```python
from build123d import *
from build123d.topology import SkipClean

# Parameters (mm, degrees)
SCHIZZO2_W            = 65.8
SCHIZZO2_H            = 15.8
FRONT_DEPTH           = 1.5
INNER_DEPTH           = 34
FRONT_CLEARANCE_DEPTH = 1
BACK_START            = -1
BACK_CLEARANCE_DEPTH  = 1
SCHIZZO7_W            = 65.8
SCHIZZO7_H            = 15.8
BACK_DEPTH            = 2
SCHIZZO9_W            = 65.8
SCHIZZO9_H            = 15.8
BACK_CLOSING_DEPTH    = 1


with BuildPart() as part:
    # Schizzo2 → Front (new, symmetric)
    with BuildSketch(Plane.XY):
        Rectangle(SCHIZZO2_W, SCHIZZO2_H)
        with BuildLine():
            Line((-27.25, 5.4), (-22.75, 5.4))
            Line((-22.75, 5.4), (-21.014451547, 2.089354811))
            ThreePointArc((-21.014451547, 2.089354811), (-25, -4.5), (-28.985548453, 2.089354811))
            Line((-28.985548453, 2.089354811), (-27.25, 5.4))
        make_face(mode=Mode.SUBTRACT)
        with BuildLine():
            Line((27.25, 5.4), (22.75, 5.4))
            Line((22.75, 5.4), (21.014451547, 2.089354811))
            ThreePointArc((21.014451547, 2.089354811), (25, -4.5), (28.985548453, 2.089354811))
            Line((28.985548453, 2.089354811), (27.25, 5.4))
        make_face(mode=Mode.SUBTRACT)
    extrude(amount=FRONT_DEPTH, both=True)

    # Schizzo5 → Inner (add)
    with SkipClean():  # the faces are left unmerged after this step: merging them gives an invalid solid
        with BuildSketch(Plane(origin=(0, 0, -1.5), x_dir=(-1, 0, 0), z_dir=(0, 0, -1))):
            with BuildLine():
                Line((-25, -7.9), (-27.35991702, -7.9))
                Line((-27.35991702, -7.9), (-28.2, -1.922498999))
                Line((-28.2, -1.922498999), (-27.5, -1.922498999))
                ThreePointArc((-27.5, -1.922498999), (-25, -2.8), (-22.5, -1.922498999))
                Line((-22.5, -1.922498999), (-21.5, -1.922498999))
                Line((-21.5, -1.922498999), (-21.5, -4.422498999))
                Line((-21.5, -4.422498999), (-21.15, -4.422498999))
                Line((-21.15, -4.422498999), (-20.726632237, -1.410080834))
                ThreePointArc((-20.726632237, -1.410080834), (-20.515143622, 0.368867555), (-21.014451547, 2.089354811))
                Line((-21.014451547, 2.089354811), (-22.75, 5.4))
                Line((-22.75, 5.4), (-27.25, 5.4))
                Line((-27.25, 5.4), (-28.985548453, 2.089354811))
                ThreePointArc((-28.985548453, 2.089354811), (-29.485161475, 0.365139069), (-29.271017396, -1.417183969))
                Line((-29.271017396, -1.417183969), (-28.35991702, -7.9))
                Line((-28.35991702, -7.9), (-32.9, -7.9))
                Line((-32.9, -7.9), (-32.9, 7.9))
                Line((-32.9, 7.9), (32.9, 7.9))
                Line((32.9, 7.9), (32.9, -7.9))
                Line((32.9, -7.9), (28.35991702, -7.9))
                Line((28.35991702, -7.9), (29.271017396, -1.417183969))
                ThreePointArc((29.271017396, -1.417183969), (29.485161475, 0.365139069), (28.985548453, 2.089354811))
                Line((28.985548453, 2.089354811), (27.25, 5.4))
                Line((27.25, 5.4), (22.75, 5.4))
                Line((22.75, 5.4), (21.014451547, 2.089354811))
                ThreePointArc((21.014451547, 2.089354811), (20.515143622, 0.368867555), (20.726632237, -1.410080834))
                Line((20.726632237, -1.410080834), (21.15, -4.422498999))
                Line((21.15, -4.422498999), (21.5, -4.422498999))
                Line((21.5, -4.422498999), (21.5, -1.922498999))
                Line((21.5, -1.922498999), (22.5, -1.922498999))
                ThreePointArc((22.5, -1.922498999), (25, -2.8), (27.5, -1.922498999))
                Line((27.5, -1.922498999), (28.2, -1.922498999))
                Line((28.2, -1.922498999), (27.35991702, -7.9))
                Line((27.35991702, -7.9), (25, -7.9))
                Line((25, -7.9), (21.638730893, -7.9))
                Line((21.638730893, -7.9), (-21.638730893, -7.9))
                Line((-21.638730893, -7.9), (-25, -7.9))
            make_face()
        extrude(amount=INNER_DEPTH)

    # Schizzo13 → Front clearance (cut)
    with BuildSketch(Plane.XY.offset(-1.5)):
        with BuildLine():
            Line((-21.5, -2.828427125), (-21.5, -4.422498999))
            Line((-21.5, -4.422498999), (-21.15, -4.422498999))
            Line((-21.15, -4.422498999), (-21.155384602, -4.46081243))
            Line((-21.155384602, -4.46081243), (-21.638730893, -7.9))
            Line((-21.638730893, -7.9), (-27.35991702, -7.9))
            Line((-27.35991702, -7.9), (-27.998629063, -3.355327665))
            Line((-27.998629063, -3.355327665), (-28.2, -1.922498999))
            Line((-28.2, -1.922498999), (-27.5, -1.922498999))
            ThreePointArc((-27.5, -1.922498999), (-25, -2.8), (-22.5, -1.922498999))
            Line((-22.5, -1.922498999), (-21.5, -1.922498999))
            Line((-21.5, -1.922498999), (-21.5, -2.828427125))
        make_face()
        with BuildLine():
            Line((21.155384602, -4.46081243), (21.638730893, -7.9))
            Line((21.638730893, -7.9), (27.35991702, -7.9))
            Line((27.35991702, -7.9), (27.998629063, -3.355327665))
            Line((27.998629063, -3.355327665), (28.2, -1.922498999))
            Line((28.2, -1.922498999), (27.5, -1.922498999))
            ThreePointArc((27.5, -1.922498999), (25, -2.8), (22.5, -1.922498999))
            Line((22.5, -1.922498999), (21.5, -1.922498999))
            Line((21.5, -1.922498999), (21.5, -2.828427125))
            Line((21.5, -2.828427125), (21.5, -4.422498999))
            Line((21.5, -4.422498999), (21.15, -4.422498999))
            Line((21.15, -4.422498999), (21.155384602, -4.46081243))
        make_face()
    extrude(amount=-FRONT_CLEARANCE_DEPTH, mode=Mode.SUBTRACT)

    # Schizzo12 → Back clearance (cut)
    with BuildSketch(Plane(origin=(0, 0, -35.5), x_dir=(-1, 0, 0), z_dir=(0, 0, -1)).offset(BACK_START)):
        with BuildLine():
            Line((21.5, -1.922498999), (21.5, -4.422498999))
            Line((21.5, -4.422498999), (21.15, -4.422498999))
            Line((21.15, -4.422498999), (21.638730893, -7.9))
            Line((21.638730893, -7.9), (27.35991702, -7.9))
            Line((27.35991702, -7.9), (28.2, -1.922498999))
            Line((28.2, -1.922498999), (27.5, -1.922498999))
            ThreePointArc((27.5, -1.922498999), (25, -2.8), (22.5, -1.922498999))
            Line((22.5, -1.922498999), (21.5, -1.922498999))
        make_face()
        with BuildLine():
            Line((-27.35991702, -7.9), (-21.638730893, -7.9))
            Line((-21.638730893, -7.9), (-21.15, -4.422498999))
            Line((-21.15, -4.422498999), (-21.5, -4.422498999))
            Line((-21.5, -4.422498999), (-21.5, -1.922498999))
            Line((-21.5, -1.922498999), (-22.5, -1.922498999))
            ThreePointArc((-22.5, -1.922498999), (-25, -2.8), (-27.5, -1.922498999))
            Line((-27.5, -1.922498999), (-28.2, -1.922498999))
            Line((-28.2, -1.922498999), (-27.35991702, -7.9))
        make_face()
    extrude(amount=BACK_CLEARANCE_DEPTH, mode=Mode.SUBTRACT)

    # Schizzo7 → Back (add)
    with BuildSketch(Plane(origin=(0, 0, -35.5), x_dir=(-1, 0, 0), z_dir=(0, 0, -1))):
        Rectangle(SCHIZZO7_W, SCHIZZO7_H)
        with BuildLine():
            Line((22.75, 5.4), (21.014451547, 2.089354811))
            ThreePointArc((21.014451547, 2.089354811), (25, -4.5), (28.985548453, 2.089354811))
            Line((28.985548453, 2.089354811), (27.25, 5.4))
            Line((27.25, 5.4), (22.75, 5.4))
        make_face(mode=Mode.SUBTRACT)
        with BuildLine():
            Line((-27.25, 5.4), (-22.75, 5.4))
            Line((-22.75, 5.4), (-21.014451547, 2.089354811))
            ThreePointArc((-21.014451547, 2.089354811), (-25, -4.5), (-28.985548453, 2.089354811))
            Line((-28.985548453, 2.089354811), (-27.25, 5.4))
        make_face(mode=Mode.SUBTRACT)
    extrude(amount=BACK_DEPTH)

    # Schizzo9 → Back closing (add)
    with BuildSketch(Plane(origin=(0, 0, -37.5), x_dir=(-1, 0, 0), z_dir=(0, 0, -1))):
        Rectangle(SCHIZZO9_W, SCHIZZO9_H)
    extrude(amount=BACK_CLOSING_DEPTH)


solid = part.part
```
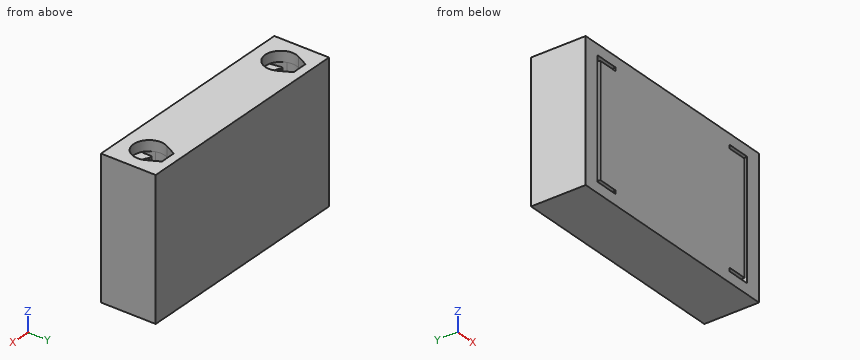
Verification items for the finished model (mm, model axes). Give positions to 0.01 mm unless a question says otherwise; leave off trailing zeros. Order: outer loops, then holes, each group sorted by start corner. A loop starts at its lowest first (then second) coordinate and runs counter-clockwise, first axis right, second up. Notation, with made-up numbers: M 41.5,-22.75 L 54.5,-22.75 A13 cw 54.5,-9.75 Z; hole C 30.5,-19 d9. An arc over 180 degrees is marked long. Return JSON: item names as keys, results as strings. Group by question number.
1) Scan lines: line 1 (X direction, y = 0, z = -0.2); line 2 (Y direction, x = -25, z = 0.65); line 3 (X direction, y = -5.25, z = -34). Record each from-to range of solid material in increasing order.
2) Section check D-D on y = 4.5. Record the cut outline in (x, z), and give its area (3 significant figures).
3) Go/stop test with a flat-tipped pin: pin 1 Ø8 at (x, y) = (25, 0) entering from +Z. Record where the tip stops, or that it passes through.
4) Section check B-B on y = 0. Record the cut outline in (x, z), and give its area (3 significant figures).
5) Section check A-A on x = 25. Record the cut outline in (y, z).
Answer block:
{
 "1": {"line 1": "x = -32.9 to -29.5, -20.5 to 20.5, 29.5 to 32.9", "line 2": "y = -7.9 to -4.5, 5.4 to 7.9", "line 3": "x = -32.9 to -28.73, -27.73 to 27.73, 28.73 to 32.9"},
 "2": {"outline": "M -32.9,-38.5 L 32.9,-38.5 L 32.9,1.5 L 27.72,1.5 L 27.72,-37.5 L 22.28,-37.5 L 22.28,1.5 L -22.28,1.5 L -22.28,-37.5 L -27.72,-37.5 L -27.72,1.5 L -32.9,1.5 Z", "area": "2,210 mm^2"},
 "3": {"pin 1": "stops at z = -2.5"},
 "4": {"outline": "M -32.9,-38.5 L 32.9,-38.5 L 32.9,1.5 L 29.5,1.5 L 29.5,-37.5 L 20.5,-37.5 L 20.5,1.5 L -20.5,1.5 L -20.5,-37.5 L -29.5,-37.5 L -29.5,1.5 L -32.9,1.5 Z", "area": "1,930 mm^2"},
 "5": {"outline": "M -7.9,-38.5 L 7.9,-38.5 L 7.9,1.5 L 5.4,1.5 L 5.4,-37.5 L -4.5,-37.5 L -4.5,-35.5 L -7.9,-35.5 Z; M -7.9,-34.5 L -2.8,-34.5 L -2.8,-2.5 L -7.9,-2.5 Z; M -7.9,-1.5 L -4.5,-1.5 L -4.5,1.5 L -7.9,1.5 Z"}
}
